Can you work these out from the model? Positions are in its coordinate system, mm. A direction names the side the tool comes from. Give positions to 0.01 mm unless a question says otherwise; leave off trailing zeros. Write each loop counter-clockwise with the first axis right and the second up, starting at its lowest first coordinate (ties: lowest second). Pieces come first, ordered by that corner, then holes.
1. I'm going to push flat-ended pins straight in: pin 1 (1 mm diameter, centred on x = -12.5, z = 3, fed in from -Y); pin 2 (4 mm diameter, centred on x = -7.5, z = 8, fed in from +Y); pin 3 (2 mm diameter, centred on y = -3, z = 1, fed in from +X). Where does each tip first touch, or does it pass through?
2. On a 3-axis mill with a long thin cutter (end or side, diameter ignored), from which of +Z, -Z, +X, -X, +Y, -Y can I reach the whole of each face in a straight line? I mean faces 5 (the cylindrical face through (5.159, 2.867, 2.465)), 6 (the flat face through (0, 12.5, 6)), 7 (the flat face through (10.775, -6.337, 6.041)), 8 (the cylindrical face through (2.214, 13.081, 2.465)). Say none if no direction works.
3. If I drill on probe 1 along X at (y, z) = (-9, 2.75); probe 2 along X at (y, z) = (4.5, 1.15); probe 3 along Y at (x, z) = (-1.5, 8), over which ranges is the centre line in solid material (lowest first)?
4. Suppose I cut it at C-C (y = -8). Please give me the cut outline in (x, z).
5. Suppose I cut it at B-B (x = 0). Please give me the cut outline in (y, z).
6. Thinking about a two-plate mould opening in Y: for faces 1 (the cylindrical face through (-11.503, 3.932, 2.465)), 2 (the flat face through (0, 0, 0)), 3 (the flat face through (-10.876, -6.163, 6.041)), 4 (the cylindrical face through (-10.19, -8.456, 2.465)), which applies, pulls with the +Y half, pulls with the -Y half, needs draft (parallel to the pull), parting line crosses it, or undercut?
7. Suppose I cut it at A-A (z = 8.5). Please give me the cut outline in (x, y), and give its area (3 significant figures).
```python
from build123d import *

# Parameters (mm, degrees)
EXTRUDE_1_DEPTH          = 10
EXTRUDE_2_DEPTH          = 5
CUT_EXTRUDE_2_DEPTH      = 5
PATTERN_CIRCULAR_1_COUNT = 3


with BuildPart() as part:
    # Sketch 1 → Extrude 1 (new body)
    with BuildSketch(Plane.XY):
        Polygon((14.43375673, 0), (7.216878365, 12.5), (-7.216878365, 12.5), (-14.43375673, 0), (-7.216878365, -12.5), (7.216878365, -12.5), align=None)
    extrude(amount=EXTRUDE_1_DEPTH)

    # Sketch 2 → Extrude 2 (add)
    with BuildSketch(Plane(origin=(0, 0, 0), x_dir=(-1, 0, 0), z_dir=(0, 0, -1))):
        with BuildLine():
            Line((-3.122498999, 12.5), (3.122498999, 12.5))
            ThreePointArc((3.122498999, 12.5), (2.22111118, 13.066987298), (2.341874249, 14.125))
            ThreePointArc((2.341874249, 14.125), (0, 19), (-2.341874249, 14.125))
            ThreePointArc((-2.341874249, 14.125), (-2.22111118, 13.066987298), (-3.122498999, 12.5))
        make_face()
    extrude_2 = extrude(amount=-EXTRUDE_2_DEPTH)

    # Sketch 3 → Cut-Extrude 2 (cut)
    with BuildSketch(Plane(origin=(0, 0, 0), x_dir=(-1, 0, 0), z_dir=(0, 0, -1))):
        with BuildLine():
            ThreePointArc((-2.457026249, -10.890243902), (-2.352465403, -11.941726104), (-3.249615362, -12.5))
            Line((-3.249615362, -12.5), (0, -12.5))
            Line((0, -12.5), (3.249615362, -12.5))
            ThreePointArc((3.249615362, -12.5), (2.352465403, -11.941726104), (2.457026249, -10.890243902))
            ThreePointArc((2.457026249, -10.890243902), (0, -5.9), (-2.457026249, -10.890243902))
        make_face()
    cut_extrude_2 = extrude(amount=-CUT_EXTRUDE_2_DEPTH, mode=Mode.SUBTRACT)

    # Pattern Circular 1: Extrude 2, Cut-Extrude 2 ×3 about axis
    pattern_circular_1_axis = Axis((0, 0, 0), (0, 0, 1))
    add([extrude_2.rotate(pattern_circular_1_axis, i * 360 / PATTERN_CIRCULAR_1_COUNT) for i in range(1, PATTERN_CIRCULAR_1_COUNT)])
    add([cut_extrude_2.rotate(pattern_circular_1_axis, i * 360 / PATTERN_CIRCULAR_1_COUNT) for i in range(1, PATTERN_CIRCULAR_1_COUNT)], mode=Mode.SUBTRACT)


solid = part.part
```
Checks:
1. pin 1: stops at y = -10.88
1. pin 2: stops at y = 12.5
1. pin 3: stops at x = 13.28
2. face 5: -Z
2. face 6: +Z, +Y
2. face 7: +Z
2. face 8: +Z, -Z, +X
3. probe 1: x = -16.68 to -11.02, -9.24 to -3.1, 3.1 to 9.24, 11.02 to 16.68
3. probe 2: x = -4.69 to 4.69
3. probe 3: y = -12.5 to 12.5
4. outline: (-16.86, 0) - (-2.93, 0) - (-2.93, 5) - (2.93, 5) - (2.93, 0) - (16.86, 0) - (16.86, 5) - (9.81, 5) - (9.81, 10) - (-9.81, 10) - (-9.81, 5) - (-16.86, 5) - close
5. outline: (-12.5, 5) - (-5.9, 5) - (-5.9, 0) - (19, 0) - (19, 5) - (12.5, 5) - (12.5, 10) - (-12.5, 10) - close
6. face 1: pulls with the +Y half
6. face 2: needs draft
6. face 3: undercut
6. face 4: pulls with the -Y half
7. outline: (-14.43, 0) - (-7.22, -12.5) - (7.22, -12.5) - (14.43, 0) - (7.22, 12.5) - (-7.22, 12.5) - close
7. area: 541 mm2
